from build123d import *

# Parameters (mm, degrees)
SKETCH_1_R          = 10
SKETCH_1_R_2        = 8.1
EXTRUDE_1_DEPTH     = 5
FILLET_1_R          = 0.2
SKETCH_3_R          = 9.1
CUT_EXTRUDE_1_DEPTH = 1


with BuildPart() as part:
    # 草图1 → 凸台-拉伸1 (new body)
    with BuildSketch(Plane(origin=(0, 0, 0), x_dir=(1, 0, 0), z_dir=(0, 1, 0))):
        Circle(SKETCH_1_R)
        Circle(SKETCH_1_R_2, mode=Mode.SUBTRACT)
    extrude(amount=EXTRUDE_1_DEPTH)

    # 草图2 → 旋转1 (revolve)
    with BuildSketch(Plane(origin=(0, 0, 0), x_dir=(0, 0, -1), z_dir=(1, 0, 0))):
        Polygon((10, 5), (10, 0), (15, 0), align=None)
    revolve(axis=Axis((0, 0, 0), (0, 1, 0)))

    # 圆角1
    fillet_1_edges = [part.edges().sort_by_distance(p)[0] for p in [
        (0, 0, 15),
    ]]
    fillet(fillet_1_edges, radius=FILLET_1_R)

    # 草图3 → 切除-拉伸1 (cut)
    with BuildSketch(Plane(origin=(0, 5, 0), x_dir=(1, 0, 0), z_dir=(0, 1, 0))):
        Circle(SKETCH_3_R)
    extrude(amount=-CUT_EXTRUDE_1_DEPTH, mode=Mode.SUBTRACT)


solid = part.part
Here's how the part is built. I have some questions about the finished solid (model axes, mm). A direction names the side the tool comes from. Coordinates: 2 decimals unless noted, no trailing zeros. Write each loop counter-clockwise with the first axis right and the second up, starting at its lowest first coordinate (ties: lowest second). Pieces come first, ordered by that corner, then holes.
1) Which directions (+Z, -Z, +X, -X, +Y, -Y) give clear straight access to the entire face, cutting with the end or side of a thin tool? Please do faces 4 (the face through (-1.973, 4.507, 8.884)), 5 (the face through (-4.5, 5, 8.1)).
Filled in:
face 4: +Y
face 5: +Z, -Z, +X, -X, +Y
2) If we section it at C-C (y = 4.6): List the corners of the cut face in (x, z) for me, plus the area to 3 significant figures.
Filled in:
outline: circle Ø20.8 at (0, 0); hole circle Ø18.2 at (0, 0)
area: 79.6 mm2
3) If we section it at A-A (z = 0): List the corners of the cut face in (x, y) for me, plus the area to 3 significant figures.
Filled in:
outline: (-14.66, 0.34) arc R0.2 ccw to (-14.52, 0) - (-8.1, 0) - (-8.1, 4) - (-9.1, 4) - (-9.1, 5) - (-10, 5) - close; (8.1, 0) - (14.52, 0) arc R0.2 ccw to (14.66, 0.34) - (10, 5) - (9.1, 5) - (9.1, 4) - (8.1, 4) - close
area: 41.9 mm2
4) I'm going to push flat-ended pins straight in: pin 1 (2 mm diameter, centred on x = 4, z = -6, fed in from +Y); pin 2 (2 mm diameter, centred on y = 3.5, z = -3.5, fed in from -X). Where does each tip first touch, or does it pass through?
Filled in:
pin 1: stops at y = 4
pin 2: stops at x = -12.04
5) If I drill on line 1 (Y direction, x = -5.25, z = -6.25); line 2 (Z direction, x = -6.25, y = 1.15); line 3 (Z direction, x = 0, y = 4.7), over which ranges is the centre line in solid material (lowest first)?
Filled in:
line 1: y = 0 to 4
line 2: z = -12.36 to -5.15, 5.15 to 12.36
line 3: z = -10.3 to -9.1, 9.1 to 10.3
6) Thinking about a two-plate mould opening in Z: for faces 1 (the face through (-1.756, 1.972, 7.907)), 2 (the face through (-3.072, 4.774, -9.754)), 3 (the face through (6, 0, 6)), which applies, +Z half, -Z half, draft (parallel to the pull), parting line (faces both ways), or undercut?
Filled in:
face 1: undercut
face 2: parting line
face 3: draft
7) If we section it at B-B (x = 0): List the corners of the cut face in (y, z) for me.
Filled in:
outline: (0, -14.52) arc R0.2 ccw to (0.34, -14.66) - (5, -10) - (5, -9.1) - (4, -9.1) - (4, -8.1) - (0, -8.1) - close; (0, 8.1) - (4, 8.1) - (4, 9.1) - (5, 9.1) - (5, 10) - (0.34, 14.66) arc R0.2 ccw to (0, 14.52) - close
